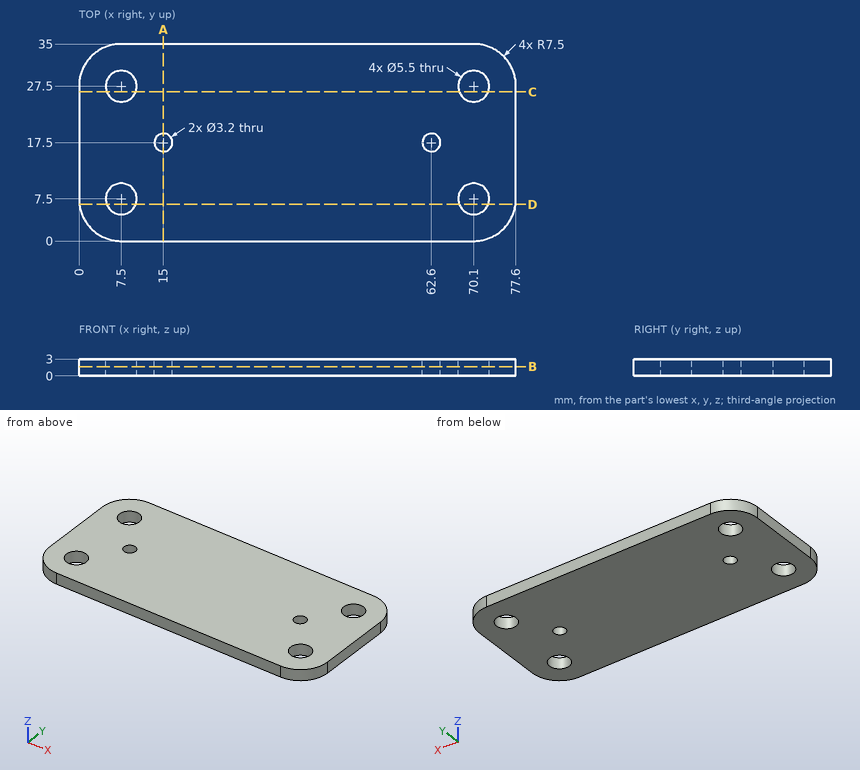
The figure shows three views and two pictorial views of one solid part (mm, origin at its lowest corner). Answer the questions. Coordinates: 2 decimals unless noted, no trailing zeros. Loops run counter-clockwise (first coordinate to the right, second up) from the corner with the lowest first, then second, coordinate; pieces in that order, holes last. Notation, with made-up numbers: (3.25, -18.75) -> (32.25, -18.75) arc R15 ccw to (32.25, 7.25) -> close; hole circle Ø7 at (-21, 71). An arc over 180 degrees is marked (long way). Write item = value, one per line. Start each with the question number.
1) A cutting plane is placed at C-C (y = 26.5). Give the vertices of the cut face in (x, z), then the cut area to 3 significant figures.
2) A cutting plane is placed at D-D (y = 6.5). Give the vertices of the cut face in (x, z).
3) A cutting plane is placed at B-B (z = 1.65). Give the vertices of the cut face in (x, y), then the cut area to 3 significant figures.
4) Straight lines are drawn through the part: line 1 (X direction, y = 27.5, z = 1.75); line 2 (Y direction, x = 7.5, z = 1.85); line 3 (X direction, y = 17.5, z = 1.05). For each, find the intervals that lie inside material, in ascending order. Write a range as from..to.
5) A cutting plane is placed at A-A (x = 15). Give the vertices of the cut face in (y, z).
6) Given pin 1 Ø5 at (x, y) = (7.5, 7.5) entering from -Z, flat-ended and moving along its own axis, determine where the tip first touches the part or whether it passes through.
Responses:
q1.outline = (0, 0) -> (4.94, 0) -> (4.94, 3) -> (0, 3) -> close; (10.06, 0) -> (67.54, 0) -> (67.54, 3) -> (10.06, 3) -> close; (72.66, 0) -> (77.6, 0) -> (77.6, 3) -> (72.66, 3) -> close
q1.area = 202 mm²
q2.outline = (0.07, 0) -> (4.94, 0) -> (4.94, 3) -> (0.07, 3) -> close; (10.06, 0) -> (67.54, 0) -> (67.54, 3) -> (10.06, 3) -> close; (72.66, 0) -> (77.53, 0) -> (77.53, 3) -> (72.66, 3) -> close
q3.outline = (0, 7.5) arc R7.5 ccw to (7.5, 0) -> (70.1, 0) arc R7.5 ccw to (77.6, 7.5) -> (77.6, 27.5) arc R7.5 ccw to (70.1, 35) -> (7.5, 35) arc R7.5 ccw to (0, 27.5) -> close; hole circle Ø5.5 at (7.5, 7.5); hole circle Ø5.5 at (7.5, 27.5); hole circle Ø3.2 at (15, 17.5); hole circle Ø3.2 at (62.6, 17.5); hole circle Ø5.5 at (70.1, 7.5); hole circle Ø5.5 at (70.1, 27.5)
q3.area = 2,560 mm²
q4.line_1 = 0..4.75, 10.25..67.35, 72.85..77.6
q4.line_2 = 0..4.75, 10.25..24.75, 30.25..35
q4.line_3 = 0..13.4, 16.6..61, 64.2..77.6
q5.outline = (0, 0) -> (15.9, 0) -> (15.9, 3) -> (0, 3) -> close; (19.1, 0) -> (35, 0) -> (35, 3) -> (19.1, 3) -> close
q6.pin_1 = through
